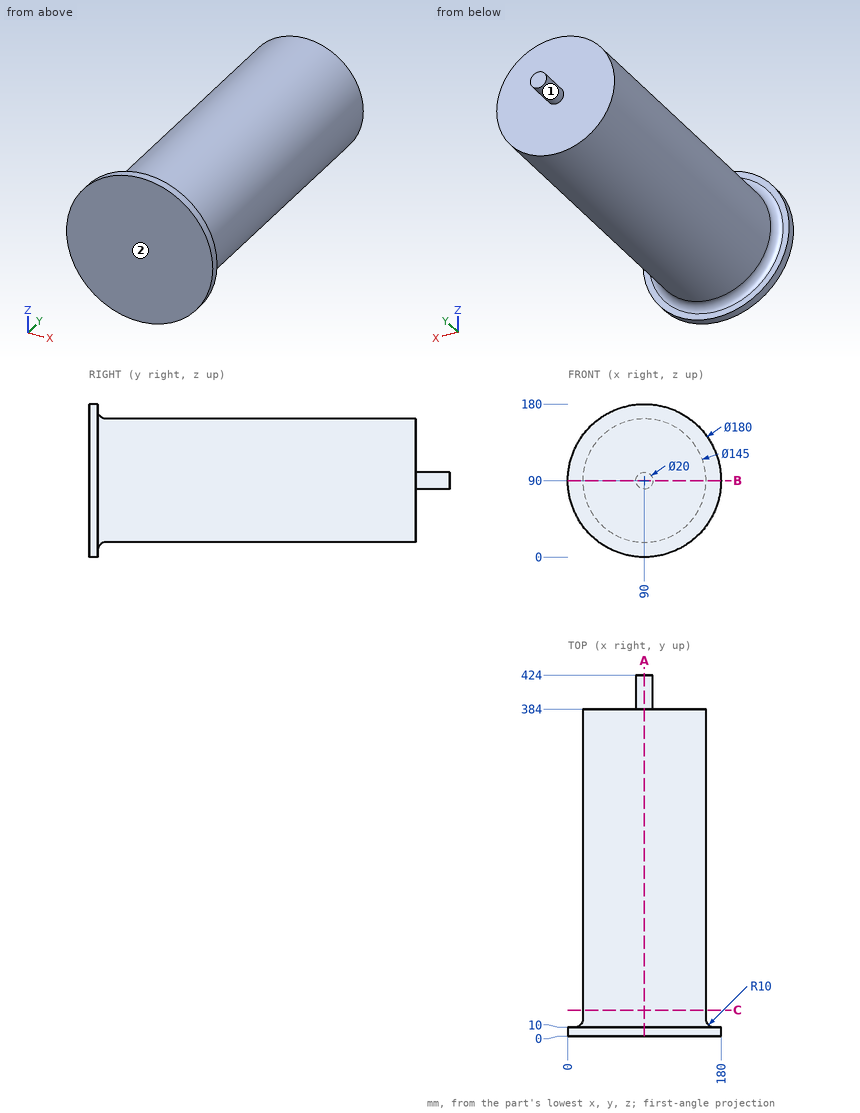
Design review of the part shown in the three views and the two pictorial views. Dimensions are in mm from the part's minimum x, y and z. A direction names the side the tool comes from. Coordinates: 2 decimals unless noted, no trailing zeros. Loops run counter-clockwise (first coordinate to the right, second up) from the corner with the lowest first, then second, coordinate; pieces in that order, holes last.
Q1. For pin 1 (1.5 mm diameter, centred on x = 82.5, y = 295, fed in from -Z); pin 2 (5 mm diameter, centred on y = 274, z = 85.5, fed in from -X); pin 3 (8 mm diameter, centred on x = 52, y = 339.5, fed in from +Z), all flat-tipped, find the tip position at first contact; note any pin that passes through.
Reported:
pin 1: stops at z = 17.81
pin 2: stops at x = 17.53
pin 3: stops at z = 154.03
Q2. To check wall thickness, follow line 1 (Y direction, x = 109, z = 150.5); line 2 (Y direction, x = 71.5, z = 17); line 3 (Z direction, x = 59.5, y = 280). State the ranges of each line that lie inside material, in increasing order.
Reported:
line 1: y = 0 to 384
line 2: y = 0 to 13.05
line 3: z = 24.23 to 155.77
Q3. We need section B-B on z = 90. State the section outline as (x, y) points, and give its area (3 significant figures).
Reported:
outline: (0, 0) - (180, 0) - (180, 10) - (172.5, 10) arc R10 cw to (162.5, 20) - (162.5, 384) - (100, 384) - (100, 424) - (80, 424) - (80, 384) - (17.5, 384) - (17.5, 20) arc R10 cw to (7.5, 10) - (0, 10) - close
area: 56,900 mm2
Q4. We need section A-A on x = 90. State the section outline as (y, z) points, and give its area (3 significant figures).
Reported:
outline: (0, 0) - (10, 0) - (10, 7.5) arc R10 cw to (20, 17.5) - (384, 17.5) - (384, 80) - (424, 80) - (424, 100) - (384, 100) - (384, 162.5) - (20, 162.5) arc R10 cw to (10, 172.5) - (10, 180) - (0, 180) - close
area: 56,900 mm2
Q5. Tool access review of the marked faces 1 and 2: name each direction out of +Z, -Z, +X, -X, +Y, -Y from which nothing blocks a thin tool from reaching the whole face with its end or side.
Reported:
face 1: +Y
face 2: +Z, -Z, +X, -X, -Y
Q6. We need section C-C on y = 30.5. State the section outline as (x, z) points, and give its area (3 significant figures).
Reported:
outline: circle Ø145 at (90, 90)
area: 16,500 mm2
